from build123d import *

# Parameters (mm, degrees)
SKETCH1_W                      = 1174.75
SKETCH1_H                      = 51.816
BASE_FLANGE1_DEPTH             = 3.2639
EDGE_FLANGE1_STRIP_W           = 17.6276
EDGE_FLANGE1_STRIP_H           = 3.2639
EDGE_FLANGE1_STRIP_CUT_DEPTH   = 1174.75
EDGE_FLANGE1_STRIP_2_W         = 17.6276
EDGE_FLANGE1_STRIP_2_H         = 3.2639
EDGE_FLANGE1_STRIP_CUT_2_DEPTH = 1174.75
EDGE_FLANGE1_DEPTH             = 1174.75
EDGE_FLANGE1_BEND_DEPTH        = 1174.75
F_10_0_1935_DIAMETER_HOLE2_D   = 4.9149
FILLET2_R                      = 6.35
F_1_4_CLEARANCE_HOLE1_D        = 6.5278


# Sheet-metal steps are written as plain solids
with BuildPart() as part:
    # Sketch1 → Base-Flange1 (new body)
    with BuildSketch(Plane(origin=(0, 0, 0), x_dir=(1, 0, 0), z_dir=(0, 1, 0))):
        Rectangle(SKETCH1_W, SKETCH1_H)
    extrude(amount=-BASE_FLANGE1_DEPTH)

    # Edge-Flange1 strip (across the edge) → Edge-Flange1 strip cut (cut)
    with BuildSketch(Plane(origin=(587.375, -3.2639, 25.908), x_dir=(0, 0, -1), z_dir=(-1, 0, 0))):
        with Locations((-6.5278, -1.63195)):
            Rectangle(EDGE_FLANGE1_STRIP_W, EDGE_FLANGE1_STRIP_H)
    extrude(amount=EDGE_FLANGE1_STRIP_CUT_DEPTH, mode=Mode.SUBTRACT)

    # Edge-Flange1 strip 2 (across the edge) → Edge-Flange1 strip cut 2 (cut)
    with BuildSketch(Plane(origin=(-587.375, -3.2639, -25.908), x_dir=(0, 0, 1), z_dir=(1, 0, 0))):
        with Locations((-6.5278, -1.63195)):
            Rectangle(EDGE_FLANGE1_STRIP_2_W, EDGE_FLANGE1_STRIP_2_H)
    extrude(amount=EDGE_FLANGE1_STRIP_CUT_2_DEPTH, mode=Mode.SUBTRACT)

    # Edge-Flange1 section (across the edge) → Edge-Flange1 (add)
    with BuildSketch(Plane(origin=(587.375, -3.2639, 25.908), x_dir=(0, 0, -1), z_dir=(-1, 0, 0))):
        with BuildLine():
            Line((-3.2639, 2.286), (-3.2639, 28.575))
            Line((-3.2639, 28.575), (0, 28.575))
            Line((0, 28.575), (0, 2.286))
            ThreePointArc((0, 2.286), (0.669553898, 0.669553898), (2.286, 0))
            Line((2.286, 0), (2.286, -3.2639))
            ThreePointArc((2.286, -3.2639), (-1.638371925, -1.638371925), (-3.2639, 2.286))
        make_face()
    extrude(amount=EDGE_FLANGE1_DEPTH)

    # Edge-Flange1 section 2 (across the edge) → Edge-Flange1 bend (add)
    with BuildSketch(Plane(origin=(-587.375, -3.2639, -25.908), x_dir=(0, 0, 1), z_dir=(1, 0, 0))):
        with BuildLine():
            Line((-3.2639, 2.286), (-3.2639, 28.575))
            Line((-3.2639, 28.575), (0, 28.575))
            Line((0, 28.575), (0, 2.286))
            ThreePointArc((0, 2.286), (0.669553898, 0.669553898), (2.286, 0))
            Line((2.286, 0), (2.286, -3.2639))
            ThreePointArc((2.286, -3.2639), (-1.638371925, -1.638371925), (-3.2639, 2.286))
        make_face()
    extrude(amount=EDGE_FLANGE1_BEND_DEPTH)

    # #10 (0.1935) Diameter Hole2 (through all)
    with Locations(Plane.XY.offset(29.1719)):
        with Locations((577.85, -22.3139), (558.8, -22.3139), (-558.8, -22.3139), (-577.85, -22.3139)):
            Hole(F_10_0_1935_DIAMETER_HOLE2_D / 2)

    # Fillet2
    fillet2_edges = [part.edges().sort_by_distance(p)[0] for p in [
        (587.375, -31.8389, 27.53995),
        (-587.375, -31.8389, 27.53995),
        (-587.375, -31.8389, -27.53995),
        (587.375, -31.8389, -27.53995),
    ]]
    fillet(fillet2_edges, radius=FILLET2_R)

    # 1/4 Clearance Hole1 (through all)
    with Locations(Plane(origin=(0, 0, 0), x_dir=(1, 0, 0), z_dir=(0, 1, 0))):
        with Locations((539.75, 0), (184.15, 0), (-184.15, 0), (-539.75, 0)):
            Hole(F_1_4_CLEARANCE_HOLE1_D / 2)


solid = part.part
Model file for the job. Use its own axes, mm. A direction names the side the tool comes from. Give positions to 0.01 mm unless a question says otherwise; leave off trailing zeros. Loops run counter-clockwise (first coordinate to the right, second up) from the corner with the lowest first, then second, coordinate; pieces in that order, holes last. Notation, with made-up numbers: (59.25, -15.75) -> (76.25, -15.75) arc R29 ccw to (76.25, 18.25) -> close; hole circle Ø3 at (-40, 55). An arc over 180 degrees is marked (long way). Use a Markdown table: item, result. Add a question column.
(1) Slice it at A-A on x = -403. List the corners of the cut face in (y, z), and give its area (3 significant figures).
(2) Slice it at B-B on z = -14.5. List the corners of the cut face in (x, y) (3 decimals).
(3) Drop a flat-ended pin along its axis: pin 1 Ø10.5 at (x, z) = (539.75, 0) entering from -Y. Give the stop position or say it passes through.
(4) Wall check: line 1 along Z through (x, y) = (538, -18.5); line 2 along Y through (x, z) = (-2, -16.5); line 3 along Y through (x, z) = (-577, -27). Give the ranges that are in metal, low to high.
(5) Tool access for faces 4 (the flat face through (-8, -3.264, 0)), 5 (the flat face through (-8, -19, -29.172)): list every direction of +Z, -Z, +X, -X, +Y, -Y with a clear straight run to the whole face (end or side of a thin tool).
(6) Mould opens along Z. For faces 1 (the flat face through (8, -19, 25.908)), 2 (the flat face through (8, -19, 29.172)), 3 (the flat face through (-8, 0, 0)) say: +Z half, -Z half, draft (parallel to the pull), parting line (faces both ways), or undercut.
Filled sheet:
| question | item | result |
|---|---|---|
| 1 | outline | (-31.84, -29.17) -> (-5.55, -29.17) arc R5.55 ccw to (0, -23.62) -> (0, 23.62) arc R5.55 ccw to (-5.55, 29.17) -> (-31.84, 29.17) -> (-31.84, 25.91) -> (-5.55, 25.91) arc R2.29 cw to (-3.26, 23.62) -> (-3.26, -23.62) arc R2.29 cw to (-5.55, -25.91) -> (-31.84, -25.91) -> close |
| 1 | area | 366 mm2 |
| 2 | outline | (-587.375, -3.264) -> (587.375, -3.264) -> (587.375, 0) -> (-587.375, 0) -> close |
| 3 | pin 1 | y = -3.26 |
| 4 | line 1 | -29.17 to -25.91, 25.91 to 29.17 |
| 4 | line 2 | -3.26 to 0 |
| 4 | line 3 | -31.84 to -24.62, -20.01 to -1.15 |
| 5 | face 4 | +X, -X, -Y |
| 5 | face 5 | -Z, +X, -X, +Y, -Y |
| 6 | face 1 | undercut |
| 6 | face 2 | +Z half |
| 6 | face 3 | draft |
